Geometry check sheet. Reference: the model listing, model coordinates, mm. Face numbers are marked on the shaded views. A direction names the side the tool comes from. Coordinates: 2 decimals unless noted, no trailing zeros. Write each loop counter-clockwise with the first axis right and the second up, starting at its lowest first coordinate (ties: lowest second). Pieces come first, ordered by that corner, then holes. Notation, with made-up numbers: (2, -28) -> (19, -28) arc R22 cw to (19, -15) -> close; hole circle Ø3 at (-4.5, 31.25). An arc over 180 degrees is marked (long way). Answer as CSV lines item,"result".
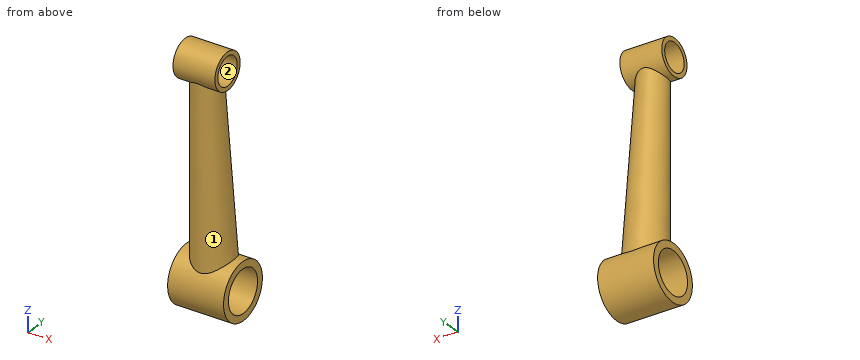
```python
from build123d import *

# Parameters (mm, degrees)
CYLINDER027_R          = 10
CYLINDER027_DEPTH      = 100
CYLINDER028_R          = 15
CYLINDER028_DEPTH      = 100
CYLINDER026_R          = 13
CYLINDER026_DEPTH      = 30
CYLINDER025_R          = 20
CYLINDER025_DEPTH      = 40
CUT015_PLACEMENT_ANGLE = 3.326608


with BuildPart() as cylinder027:
    # Cylinder027 → Cylinder027 (new body)
    with BuildSketch(Plane(origin=(50, 0, 150), x_dir=(0, 0, 1), z_dir=(-1, 0, 0))):
        Circle(CYLINDER027_R)
    extrude(amount=CYLINDER027_DEPTH)


with BuildPart() as compound010:
    # Cylinder028 → Cylinder028 (new body)
    with BuildSketch(Plane.ZY.offset(-50)):
        Circle(CYLINDER028_R)
    extrude(amount=CYLINDER028_DEPTH)

    # Compound010: union Cylinder027
    add(cylinder027.part)


with BuildPart() as cone005:
    # Cone001004 → Cone001004 (revolve)
    with BuildSketch(Plane.XZ):
        Polygon((0, 0), (15, 0), (10, 150), (0, 150), align=None)
    revolve(axis=Axis((0, 0, 0), (0, 0, 1)))


with BuildPart() as cylinder026:
    # Cylinder026 → Cylinder026 (new body)
    with BuildSketch(Plane(origin=(15, 0, 150), x_dir=(0, 0, 1), z_dir=(-1, 0, 0))):
        Circle(CYLINDER026_R)
    extrude(amount=CYLINDER026_DEPTH)


with BuildPart() as crank002:
    # Cylinder025 → Cylinder025 (new body)
    with BuildSketch(Plane.ZY.offset(-20)):
        Circle(CYLINDER025_R)
    extrude(amount=CYLINDER025_DEPTH)

    # Fusion003002003004006: union Cone005, Cylinder026
    add(cone005.part)
    add(cylinder026.part)

    # Cut015: cut Compound010
    add(compound010.part, mode=Mode.SUBTRACT)


with BuildPart() as crank002_1:
    # Cut015 placement: moved
    add(crank002.part.moved(Location((200, 8.704146, -33.900411))).rotate(Axis((200, 8.704146, -33.900411), (1, 0, 0)), CUT015_PLACEMENT_ANGLE))


solid = crank002_1.part
```
Item 1: Cross-section at D-D, the plane y = 25.5. Record the cut outline in (x, z).
Responses:
outline,"(180, -44.76) -> (220, -44.76) -> (220, -23.04) -> (180, -23.04) -> close"
Item 2: Thickness scan on probe 1 along Z at (x, y) = (210, -7.5); probe 2 along Z at (x, y) = (198, 0); probe 3 along Y at (x, z) = (189.5, -33). Record the ranges inside material, lowest first.
Responses:
probe 1,"z = -45.62 to -22.18, 105.23 to 109.23, 122.46 to 126.47"
probe 2,"z = -51.91 to -46.12, -21.68 to 105.85, 125.85 to 128.85"
probe 3,"y = -11.28 to -6.27, 23.68 to 28.68"
Item 3: Depth check by flat-ended pin: pin 1 Ø18 at (y, z) = (8.7, -33.9) entering from +X; pin 2 Ø5 at (x, z) = (213.5, -25) entering from -Y; pin 3 Ø1.5 at (x, z) = (198, 6.5) entering from +Y; pin 4 Ø4 at (x, z) = (210.5, 102.5) entering from +Y. Enter the tip coordinate at first touch or a pass-through.
Responses:
pin 1,"passes through"
pin 2,"stops at y = -10.24"
pin 3,"stops at y = 20.03"
pin 4,"stops at y = 6.89"
Item 4: Set-up check for the marked faces 1 and 2: record each of +Z, -Z, +X, -X, +Y, -Y from which the full face is reachable in a straight line by a thin tool's end or side.
Responses:
face 1,"none"
face 2,"+X, -X"
Item 5: Cross-section at A-A, the plane y = 2.5. Count the separate pieces of the cut face and the enclosed holes in it, plus the area to 3 significant figures.
Responses:
separate pieces,"3"
enclosed holes,"0"
area,"3,480 mm2"
